Could you check a few things on this model? Use its own coordinates, in mm. Face numbers are marked on the shaded views. A direction names the side the tool comes from. Give positions to 0.01 mm unless a question says otherwise; leave off trailing zeros. Write each loop counter-clockwise with the first axis right and the second up, starting at its lowest first coordinate (ties: lowest second). Pieces come first, ordered by that corner, then holes. Notation, with made-up numbers: (-6, 0) - (26, 0) arc R20 cw to (26, 25) - close; hole circle Ø3 at (-13.75, 32.5). An arc over 180 degrees is marked (long way). Answer as CSV lines item,"result". Start each with the question number.
Q1. Imagine slicing it at A-A on x = 16. List the corners of the cut face in (y, z) for me.
Q2. On a 3-axis mill with a long thin cutter (end or side, diameter ignored), from which of +Z, -Z, +X, -X, +Y, -Y can I reach the whole of each face in a straight line? I mean the marked faces 1, 2 and 3. Say none if no direction works.
Q3. Will these pins go through, and if not, where does the flat tip stop? pin 1 Ø3 at (y, z) = (-19, 29.5) entering from +X; pin 2 Ø6 at (x, y) = (0, -12.55) entering from -Z; pin 3 Ø10 at (y, z) = (-22, -10) entering from +X.
Q4. Imagine slicing it at B-B on x = 0. List the corners of the cut face in (y, z) for me (3 decimals), and give its area (3 significant figures).
Q5. Imagine slicing it at C-C on z = -26. List the corners of the cut face in (x, y) for me.
Q6. We'd pull the mould along X, two halves only. Please class the marked faces 4, 5 and 6: pulls with the +X half, pulls with the -X half, needs draft (parallel to the pull), parting line crosses it, or undercut.
Q7. If I drill on line 1 along Z through (x, y) = (-21.5, -16.5) (3 decimals); line 2 along X through (y, z) = (-13.75, -5.5); line 3 along Z through (x, y) = (1, -2) (3 decimals), over which ranges is the centre line in solid material (lowest first)?
```python
from build123d import *

# Parameters (mm, degrees)
F1_DEPTH  = 7.5
F2_DEPTH  = 17.6
F4_DEPTH  = 7.5
F6_DEPTH  = 25
F7_DEPTH  = 25.1
F8_R      = 2.5
F9_DEPTH  = 121.4
F10_DEPTH = 25.1
F11_R     = 6
F11_R_2   = 2.5
F12_DEPTH = 82
F14_DEPTH = 25.1


# Not quite as in the source:
# - a feature names something its author has since deleted; it is built from what else it names


with BuildPart() as f1:
    # F0 (on Front) → F1 (new body)
    with BuildSketch(Plane.XZ):
        with BuildLine():
            Line((24.609375, 40.625), (-25.390625, 40.625))
            Line((-25.390625, 40.625), (-25.390625, 31.7128804606))
            ThreePointArc((-25.390625, 31.7128804606), (-31.7255791152, 25.3747562511), (-36.5168539326, 17.8019662921))
            ThreePointArc((-36.5168539326, 17.8019662921), (-11.5217513517, -38.9568976022), (40.3254101185, -4.924624227))
            Line((40.3254101185, -4.924624227), (31.6393058234, -4.924624227))
            ThreePointArc((31.6393058234, -4.924624227), (-30.8610352871, -8.5378040369), (24.609375, 20.4860015345))
            Line((24.609375, 20.4860015345), (24.609375, 32.3228910698))
            Line((24.609375, 32.3228910698), (24.609375, 40.625))
        make_face()
        with BuildLine():
            Line((31.6393058234, -4.924624227), (40.3254101185, -4.924624227))
            ThreePointArc((40.3254101185, -4.924624227), (40.5500333604, -2.4668642988), (40.625, 0))
            ThreePointArc((40.625, 0), (36.3226342652, -4.3023657348), (32.0202685305, 0))
            ThreePointArc((32.0202685305, 0), (31.9248857895, -2.469668822), (31.6393058234, -4.924624227))
        make_face()
        with BuildLine():
            Line((38.6976342652, 0), (40.625, 0))
            ThreePointArc((40.625, 0), (36.3226342652, 4.3023657348), (32.0202685305, 0))
            Line((32.0202685305, 0), (33.9476342652, 0))
            ThreePointArc((33.9476342652, 0), (36.3226342652, 2.375), (38.6976342652, 0))
        make_face()
        with BuildLine():
            ThreePointArc((32.0202685305, 0), (36.3226342652, -4.3023657348), (40.625, 0))
            Line((40.625, 0), (38.6976342652, 0))
            ThreePointArc((38.6976342652, 0), (36.3226342652, -2.375), (33.9476342652, 0))
            Line((33.9476342652, 0), (32.0202685305, 0))
        make_face()
    extrude(amount=F1_DEPTH)

    # F0 (on Front) → F2 (join)
    with BuildSketch(Plane.XZ):
        with BuildLine():
            Line((24.609375, 40.625), (-25.390625, 40.625))
            Line((-25.390625, 40.625), (-25.390625, 31.7128804606))
            ThreePointArc((-25.390625, 31.7128804606), (-31.7255791152, 25.3747562511), (-36.5168539326, 17.8019662921))
            ThreePointArc((-36.5168539326, 17.8019662921), (-11.5217513517, -38.9568976022), (40.3254101185, -4.924624227))
            Line((40.3254101185, -4.924624227), (31.6393058234, -4.924624227))
            ThreePointArc((31.6393058234, -4.924624227), (-30.8610352871, -8.5378040369), (24.609375, 20.4860015345))
            Line((24.609375, 20.4860015345), (24.609375, 32.3228910698))
            Line((24.609375, 32.3228910698), (24.609375, 40.625))
        make_face()
    extrude(amount=F2_DEPTH)

    # F3 (on face) → F4 (join)
    with BuildSketch(Plane.XZ.offset(17.6)):
        with BuildLine():
            Line((24.609375, 40.625), (-25.390625, 40.625))
            Line((-25.390625, 40.625), (-25.390625, 31.7128804606))
            ThreePointArc((-25.390625, 31.7128804606), (-19.7822809369, -35.4831225505), (40.3254101185, -4.924624227))
            Line((40.3254101185, -4.924624227), (31.6393058234, -4.924624227))
            ThreePointArc((31.6393058234, -4.924624227), (-30.8610352871, -8.5378040369), (24.609375, 20.4860015345))
            Line((24.609375, 20.4860015345), (24.609375, 32.3228910698))
            Line((24.609375, 32.3228910698), (24.609375, 40.625))
        make_face()
        with BuildLine():
            Line((31.6393058234, -4.924624227), (40.3254101185, -4.924624227))
            ThreePointArc((40.3254101185, -4.924624227), (40.5500333604, -2.4668642988), (40.625, 0))
            ThreePointArc((40.625, 0), (36.3226342652, -4.3023657348), (32.0202685305, 0))
            ThreePointArc((32.0202685305, 0), (31.9248857895, -2.469668822), (31.6393058234, -4.924624227))
        make_face()
        with BuildLine():
            ThreePointArc((32.0202685305, 0), (36.3226342652, -4.3023657348), (40.625, 0))
            Line((40.625, 0), (38.6976342652, 0))
            ThreePointArc((38.6976342652, 0), (36.3226342652, -2.375), (33.9476342652, 0))
            Line((33.9476342652, 0), (32.0202685305, 0))
        make_face()
        with BuildLine():
            Line((38.6976342652, 0), (40.625, 0))
            ThreePointArc((40.625, 0), (36.3226342652, 4.3023657348), (32.0202685305, 0))
            Line((32.0202685305, 0), (33.9476342652, 0))
            ThreePointArc((33.9476342652, 0), (36.3226342652, 2.375), (38.6976342652, 0))
        make_face()
    extrude(amount=F4_DEPTH)

    # F5 (on face) → F6 (join)
    with BuildSketch(Plane.XZ.offset(25.1)):
        with BuildLine():
            Line((-24.609375, 20.4860015345), (24.609375, 20.4860015345))
            ThreePointArc((24.609375, 20.4860015345), (0, 32.0202685305), (-24.609375, 20.4860015345))
        make_face()
    extrude(amount=-F6_DEPTH)

    # F0 (on Front) → F7 (join)
    with BuildSketch(Plane.XZ):
        with BuildLine():
            Line((33.9476342652, 0), (38.6976342652, 0))
            ThreePointArc((38.6976342652, 0), (36.3226342652, 2.375), (33.9476342652, 0))
        make_face()
        with BuildLine():
            ThreePointArc((33.9476342652, 0), (36.3226342652, -2.375), (38.6976342652, 0))
            Line((38.6976342652, 0), (33.9476342652, 0))
        make_face()
    extrude(amount=F7_DEPTH)

    # F8 (on face) → F9 (cut)
    with BuildSketch(Plane.XY.offset(40.625)):
        with Locations((0, -12.55)):
            Circle(F8_R)
    extrude(amount=-F9_DEPTH, mode=Mode.SUBTRACT)

    # F0 (on Front) → F10 (join)
    with BuildSketch(Plane.XZ):
        with BuildLine():
            Line((-25.390625, 31.7128804606), (-25.390625, 40.625))
            Line((-25.390625, 40.625), (-36.5168539326, 17.8019662921))
            ThreePointArc((-36.5168539326, 17.8019662921), (-31.7255791152, 25.3747562511), (-25.390625, 31.7128804606))
        make_face()
    extrude(amount=F10_DEPTH)

    # F11 (on face) → F12 (cut)
    with BuildSketch(Plane(origin=(0, 0, 20.4860015345), x_dir=(1, 0, 0), z_dir=(0, 0, -1))):
        with Locations((0, 12.55)):
            Circle(F11_R)
        with Locations((0, 12.55)):
            Circle(F11_R_2, mode=Mode.SUBTRACT)
    extrude(amount=F12_DEPTH, mode=Mode.SUBTRACT)

    # F13 (on face) → F14 (cut)
    with BuildSketch(Plane.XZ.offset(25.1)):
        with BuildLine():
            ThreePointArc((23.1832968576, 29.9158197188), (23.3145518173, 30.2237646688), (23.359375, 30.5555007673))
            ThreePointArc((23.359375, 30.5555007673), (22.109375, 31.8055007673), (20.859375, 30.5555007673))
            ThreePointArc((20.859375, 30.5555007673), (21.7776389015, 29.35032395), (23.1832968576, 29.9158197188))
        make_face()
        with BuildLine():
            Line((24.085752666, 30.5555007673), (23.359375, 30.5555007673))
            ThreePointArc((23.359375, 30.5555007673), (23.3145518173, 30.2237646688), (23.1832968576, 29.9158197188))
            Line((23.1832968576, 29.9158197188), (24.085752666, 30.5555007673))
        make_face()
        with BuildLine():
            ThreePointArc((20.859375, 30.5555007673), (22.109375, 31.8055007673), (23.359375, 30.5555007673))
            Line((23.359375, 30.5555007673), (24.085752666, 30.5555007673))
            Line((24.085752666, 30.5555007673), (24.609375, 30.5555007673))
            Line((24.609375, 30.5555007673), (24.609375, 40.625))
            Line((24.609375, 40.625), (15.0185888633, 40.625))
            Line((15.0185888633, 40.625), (20.859375, 30.5555007673))
        make_face()
    extrude(amount=-F14_DEPTH, mode=Mode.SUBTRACT)


solid = f1.part
```
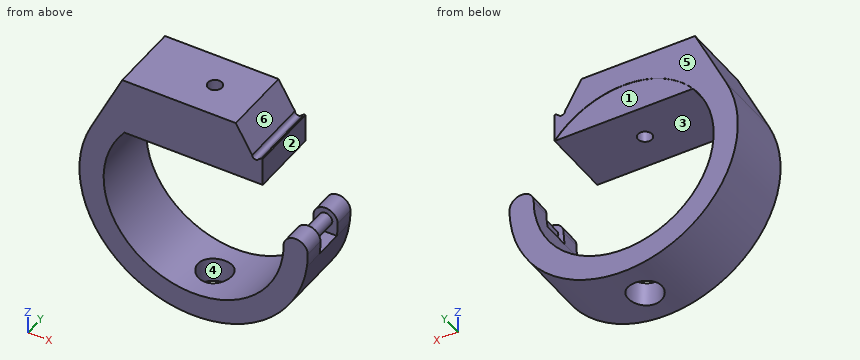
Conclusion:
1,outline,"(-25.1, -37.34) - (0, -37.34) - (0, -27.74) - (-25.1, -27.74) - close; (-25.1, 20.49) - (-0.1, 20.49) - (-0.1, 27.74) - (0, 27.74) - (0, 38.93) - (-25.1, 38.93) - close"
2,face 1,"+Y"
2,face 2,"+Z, +X, +Y, -Y"
2,face 3,"+X, +Y, -Y"
3,pin 1,"x = 24.61"
3,pin 2,"z = 20.49"
3,pin 3,"x = 40.32"
4,outline,"(-25.1, -40.625) - (-18.55, -40.625) - (-18.55, -32.02) - (-25.1, -32.02) - close; (-25.1, 20.486) - (-15.05, 20.486) - (-15.05, 40.625) - (-25.1, 40.625) - close; (-10.05, 20.486) - (-0.1, 20.486) - (-0.1, 32.02) - (0, 32.02) - (0, 40.625) - (-10.05, 40.625) - close; (-6.55, -40.625) - (0, -40.625) - (0, -32.02) - (-6.55, -32.02) - close"
4,area,"516 mm^2"
5,outline,"(-31.22, -25.1) - (-18.69, -25.1) - (-18.69, 0) - (-31.22, 0) - close; (18.69, -25.1) - (31.22, -25.1) - (31.22, 0) - (18.69, 0) - close"
6,face 4,"undercut"
6,face 5,"needs draft"
6,face 6,"pulls with the +X half"
7,line 1,"-34.469 to -23.729, 20.486 to 40.625"
7,line 2,"-40.25 to -31.54, 31.54 to 40.25"
7,line 3,"-40.613 to -32.005, 20.486 to 40.625"
